Autodesk Inventor part; units mm, degrees
ref_plane "YZ Plane" through (0, 0, 0) normal (1, 0, 0) x (0, 1, 0)
ref_plane "XZ Plane" through (0, 0, 0) normal (0, 1, 0) x (-1, 0, 0)
ref_plane "XY Plane" through (0, 0, 0) normal (0, 0, 1) x (1, 0, 0)
sketch "Sketch_1" plane through (0, 0, 0) normal (0, 0, 1) x (1, 0, 0)
  line L0 (6, 0) -> (0, 0)
  line L1 (0, 0) -> (0, 2.75)
  line L2 (0, 2.75) -> (0.1072, 3.15)
  line L3 (0.1072, 3.15) -> (5.8928, 3.15)
  line L4 (5.8928, 3.15) -> (6, 2.75)
  line L5 (6, 2.75) -> (6, 0)
  line L6 (6, 0) -> (0, 0)
revolve "Revolution1" add sketch "Sketch_1" angle 360 about axis through (6, 0, 0) along (1, 0, 0)
sketch "Sketch_5" plane through (0, 0, 0) normal (0, 0, 1) x (1, 0, 0)
  line L0 (0, 0) -> (-6, 0)
  line L1 (-6, 0) -> (-6, 1.1935)
  line L2 (-6, 1.1935) -> (-5.6935, 1.5)
  line L3 (-5.6935, 1.5) -> (-0.6, 1.5)
  line L4 (-0.6, 1.5) -> (-0.6, 1.2295)
  line L5 (-0.6, 1.2295) -> (0, 1.2295)
  line L6 (0, 1.2295) -> (0, 0)
  line L7 (0, 0) -> (-6, 0)
revolve "Revolution2" add sketch "Sketch_5" angle 360 about axis through (0, 0, 0) along (1, 0, 0)
thread "Thread1"
sketch "Sketch_6" plane through (0, 0, 0) normal (1, 0, 0) x (0, 1, 0)
  circle A0 centre (0, 0) radius 6.3
  line L0 (1.5877, 2.75) -> (-1.5877, 2.75)
  line L1 (-1.5877, 2.75) -> (-3.1754, 0)
  line L2 (-3.1754, 0) -> (-1.5877, -2.75)
  line L3 (-1.5877, -2.75) -> (1.5877, -2.75)
  line L4 (1.5877, -2.75) -> (3.1754, 0)
  line L5 (3.1754, 0) -> (1.5877, 2.75)
extrude "Extrusion1" cut sketch "Sketch_6" along normal blind 6
sketch "Sketch4" plane through (6, 0, 0) normal (1, 0, 0) x (0, 0, -1)
  point P0 (0, 0)
hole "Hole1" at (6, 0, 0) direction (-1, 0, 0) diameter 2.459 depth 4.0901 tip angle 120 countersink diameter 3 countersink angle 90
sketch "スケッチ5" plane through (-6, 0, 0) normal (-1, 0, 0) x (0, 0, 1)
  circle A0 centre (0, 0) radius 1.1935
  circle A1 centre (0, 0) radius 1.2
  circle A2 centre (0, 0) radius 2.1125
  dimension "d13" = 2.4
extrude "押し出し2" cut sketch "スケッチ5" against normal blind 6 contours A2
sketch "スケッチ6" plane through (-6, 0, 0) normal (-1, 0, 0) x (0, 0, 1)
  circle A0 centre (0, 0) radius 1.1935
  circle A1 centre (0, 0) radius 4.3291
extrude "押し出し3" cut sketch "スケッチ6" against normal blind 3 contours A0 | A1
properties part number "SLCG5.5-6"
Verification items for the finished model (mm, model axes). A direction names the side the tool comes from. Give positions to 0.01 mm unless a question says otherwise; leave off trailing zeros. Order: outer loops, then holes, each group sorted by start corner. A loop starts at its lowest first (then second) coordinate and runs counter-clockwise, first axis right, second up. Notation, with made-up numbers: M 4.5,-2.5 L 10.5,-2.5 A35 cw 10.5,33.5 Z; hole C 10.5,54 d1. An arc over 180 degrees is marked long. Answer as a JSON object with one key per item and string values. Group by question number.
1) Mould release check, pull along Y, two halves, no side actions. Record for faces 3 (the face through (6, 1.2, -1.2)), 4 (the face through (1.323, -0.208, 0.046)), 5 (the face through (0.046, 1.45, -2.536)), 6 (the face through (2.96, -2.39, -1.36)): released by +Y, released by -Y, zero draft, split by the parting line, or undercut.
2) Cross-section at D-D (x = -1.5). Enter the section's corners in (y, z), then the cut area to 3 significant figures.
3) Cross-section at C-C (x = 1.75). Enter the section's corners in (y, z).
4) Access from +Z, -Z, +X, -X, +Y, -Y to the whole of each face (thin tool, end or side, straight path). Record for faces 1 (the face through (-1.52, 1.01, 0.65)), 2 (the face through (5.95, -1.47, 2.54)).
5) Cross-section at A-A (x = 3.5). Enter the section's corners in (y, z).
6) Scan lines: line 1 along Y through (x, z) = (4.7, 0); line 2 along Z through (x, y) = (3.3, 0); line 3 along X through (y, z) = (2.5, -0.55). Record each from-to range of solid material in increasing order. Write a range as [from, to].
7) Cross-section at B-B (x = 0.5). Enter the section's corners in (y, z).
8) Depth check by flat-ended pin: pin 1 Ø2 at (x, z) = (1.5, 1.5) entering from -Y; pin 2 Ø1.5 at (x, z) = (-1.5, -1.5) entering from +Y; pin 3 Ø2 at (y, z) = (2, 2) entering from -X. Enter the tip coordinate at first touch or a pass-through.
Result sheet:
{
 "1": {"face 3": "zero draft", "face 4": "undercut", "face 5": "released by +Y", "face 6": "released by -Y"},
 "2": {"outline": "C 0,0 d2.4", "area": "4.52 mm2"},
 "3": {"outline": "M -3.15,-0.04 L -1.61,-2.71 A3.15 ccw -1.54,-2.75 L 1.54,-2.75 A3.15 ccw 1.61,-2.71 L 3.15,-0.04 A3.15 ccw 3.15,0.04 L 1.61,2.71 A3.15 ccw 1.54,2.75 L -1.54,2.75 A3.15 ccw -1.61,2.71 L -3.15,0.04 A3.15 ccw Z; hole C 0,0 d1.91"},
 "4": {"face 1": "-X", "face 2": "+Z, +X, -Y"},
 "5": {"outline": "M -3.15,-0.04 L -1.61,-2.71 A3.15 ccw -1.54,-2.75 L 1.54,-2.75 A3.15 ccw 1.61,-2.71 L 3.15,-0.04 A3.15 ccw 3.15,0.04 L 1.61,2.71 A3.15 ccw 1.54,2.75 L -1.54,2.75 A3.15 ccw -1.61,2.71 L -3.15,0.04 A3.15 ccw Z; hole C 0,0 d2.46"},
 "6": {"line 1": "y = [-3.15, -1.23], [1.23, 3.15]", "line 2": "z = [-2.75, -1.23], [1.23, 2.75]", "line 3": "x = [0, 6]"},
 "7": {"outline": "M -3.15,-0.04 L -1.61,-2.71 A3.15 ccw -1.54,-2.75 L 1.54,-2.75 A3.15 ccw 1.61,-2.71 L 3.15,-0.04 A3.15 ccw 3.15,0.04 L 1.61,2.71 A3.15 ccw 1.54,2.75 L -1.54,2.75 A3.15 ccw -1.61,2.71 L -3.15,0.04 A3.15 ccw Z"},
 "8": {"pin 1": "stops at y = -2.89", "pin 2": "stops at y = 0.94", "pin 3": "stops at x = 0"}
}
